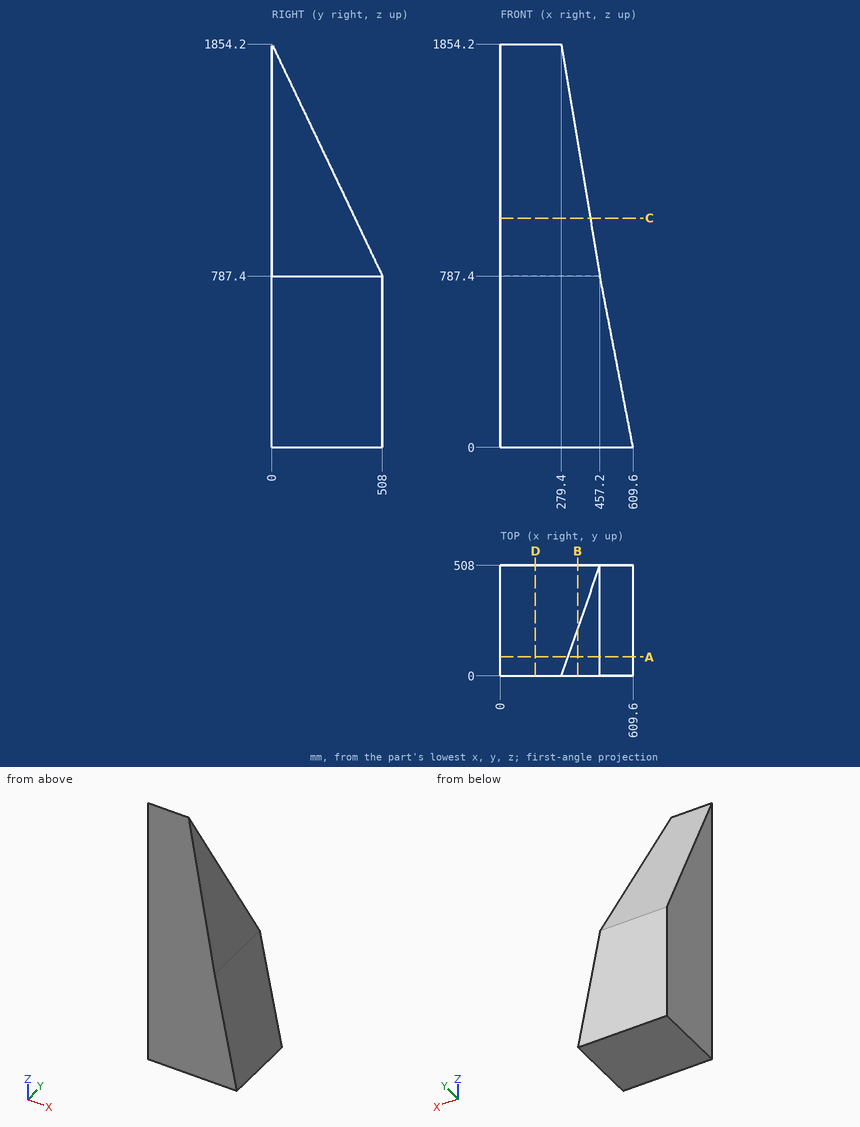
Could you check a few things on this drawing? It's one solid part, dimensions in mm from its lowest x, y, z. Coordinates: 2 decimals unless noted, no trailing zeros. Order: outer loops, then holes, each group sorted by start corner. A loop starts at its lowest first (then second) coordinate and runs counter-clockwise, first axis right, second up. Notation, with made-up numbers: M 31,80 L 81,80 A32 ccw 81,106 Z; hole C -32,-23 d6. An arc over 180 degrees is marked long. Use one line per item in the form item = value. Start each with the question number.
1. Suppose I cut it at A-A on y = 88. Write out the boundary of the cut face in (x, z).
2. For pin 1 (1.5 mm diameter, centred on x = 123.5, z = 1304.5, fed in from +Y); pin 2 (10 mm diameter, centred on y = 115, z = 1468, fed in from +X); pin 3 (8 mm diameter, centred on x = 347.5, z = 902, fed in from +Y); pin 4 (1 mm diameter, centred on x = 197.5, y = 245, fed in from -Z), each with a flat end and sliding along its axis, tell me the tip position at first contact or that it passes through.
3. Please list where these lines run through material, in increasing order: line 1 (Y direction, x = 349, z = 1396); line 2 (Z direction, x = 263.5, y = 424); line 3 (Y direction, x = 176, z = 1461.5).
4. Suppose I cut it at D-D on x = 160. Write out the boundary of the cut face in (y, z), then the cut area to 3 significant figures.
5. Suppose I cut it at C-C on z = 1053.5. Write out the boundary of the cut face in (x, y).
6. Suppose I cut it at B-B on x = 355. Write out the boundary of the cut face in (y, z).
Geometry says:
q1.outline = M 0,0 L 609.6,0 L 457.2,787.4 L 310.2,1669.4 L 0,1669.4 Z
q2.pin_1 = 262.12
q2.pin_2 = 344.6
q2.pin_3 = 455.33
q2.pin_4 = 0
q3.line_1 = 0 to 218.19
q3.line_2 = 0 to 963.8
q3.line_3 = 0 to 187
q4.outline = M 0,0 L 508,0 L 508,787.4 L 0,1854.2 Z
q4.area = 671,000 mm^2
q5.outline = M 0,0 L 412.85,0 L 412.85,381.29 L 0,381.29 Z
q6.outline = M 0,0 L 508,0 L 508,787.4 L 216,1400.6 L 0,1400.6 Z
